The listing builds one solid part. Answer for the finished solid, in the listing's coordinates (mm). Face numbers are marked on the shaded views. A direction names the side the tool comes from. Give positions to 0.01 mm unless a question says otherwise; leave off trailing zeros. Loops run counter-clockwise (first coordinate to the right, second up) from the corner with the lowest first, then second, coordinate; pieces in that order, holes last. Notation, with made-up numbers: (51.5, 31.5) - (75.5, 31.5) arc R19 ccw to (75.5, 63.5) - close; hole circle Ø7 at (-11.75, 51.25). An arc over 180 degrees is marked (long way). Write item = value, one per line. Start each with the question number.
1) Which of the six approach directions +Z, -Z, +X, -X, +Y, -Y give full straight-line access (tool end or side, diameter ignored) to the marked faces 1 and 2?
2) Flat-ended cylindrical pins translate along their axes: P1, Ø3.5, axis at x = 49.5, y = -12.5, coming from the +Z side; P2, Ø2.5, axis at y = -20.5, z = 44.6, coming from the +X side; P3, Ø12, axis at y = -5, z = 23.5, coming from the -X side. Find the tip coordinate at first contact, or state that the pin passes through.
3) The part is cut by section A-A on z = 44.6. Write down the section's boundary in (x, y), plus the area to 3 significant figures.
4) The part is cut by section D-D on y = -20.5. Write down the section's boundary in (x, z).
5) The part is cut by section C-C on y = -12.5. Write down the section's boundary in (x, z), plus the area to 3 significant figures.
6) Consider probe 1 along Y at (x, z) = (57.5, 1); probe 2 along X at (y, z) = (-20.5, 0.9); probe 3 along Y at (x, z) = (101.25, 36.6). Determine where each line is inside the solid, lowest interval first.
7) The part is cut by section B-B on x = 57.5. Write down the section's boundary in (y, z).
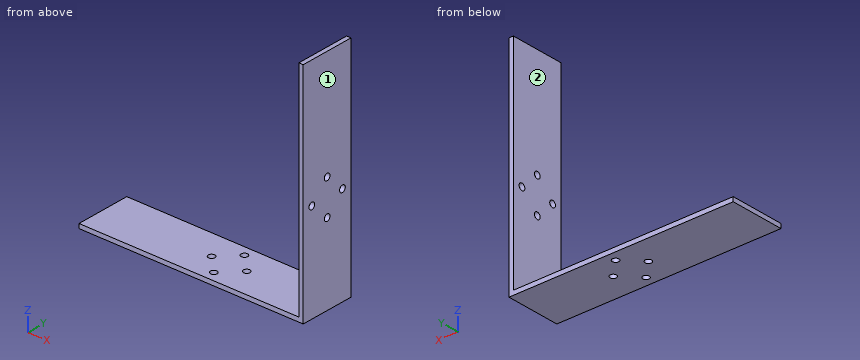
from build123d import *

# Parameters (mm, degrees)
BOSS_EXTRUDE1_DEPTH = 25
SKETCH2_R           = 1.5
CUT_EXTRUDE1_DEPTH  = 11.313708668
SKETCH3_R           = 1.5
CUT_EXTRUDE2_DEPTH  = 25


with BuildPart() as part:
    # Sketch1 → Boss-Extrude1 (new body)
    with BuildSketch(Plane(origin=(0, 0, 0), x_dir=(1, 0, 0), z_dir=(0, 1, 0))):
        Polygon((0, 0), (102.1, 0), (102.1, -102.1), (100.1, -102.1), (100.1, -2), (0, -2), align=None)
    extrude(amount=-BOSS_EXTRUDE1_DEPTH)

    # Sketch2 → Cut-Extrude1 (cut)
    with BuildSketch(Plane(origin=(0, 0, 0), x_dir=(-1, 0, 0), z_dir=(0, 0, -1))):
        with Locations((-65.500000119, -12.5)):
            Circle(SKETCH2_R)
        with Locations((-57.5, -20.500000119)):
            Circle(SKETCH2_R)
        with Locations((-49.499999881, -12.5)):
            Circle(SKETCH2_R)
        with Locations((-57.5, -4.499999881)):
            Circle(SKETCH2_R)
    extrude(amount=-CUT_EXTRUDE1_DEPTH, mode=Mode.SUBTRACT)

    # Sketch3 → Cut-Extrude2 (cut)
    with BuildSketch(Plane(origin=(102.1, 0, 0), x_dir=(0, 0, -1), z_dir=(1, 0, 0))):
        with Locations((-44.6, -4.499999881)):
            Circle(SKETCH3_R)
        with Locations((-36.599999881, -12.5)):
            Circle(SKETCH3_R)
        with Locations((-52.600000119, -12.5)):
            Circle(SKETCH3_R)
        with Locations((-44.6, -20.500000119)):
            Circle(SKETCH3_R)
    extrude(amount=-CUT_EXTRUDE2_DEPTH, mode=Mode.SUBTRACT)


solid = part.part
Answer below:
q1.face_1 = +Z, -Z, +X, +Y, -Y
q1.face_2 = +Z, -X, +Y, -Y
q2.P1 = 2
q2.P2 = through
q2.P3 = 100.1
q3.outline = (100.1, -25) - (102.1, -25) - (102.1, -22) - (100.1, -22) - close; (100.1, -19) - (102.1, -19) - (102.1, -6) - (100.1, -6) - close; (100.1, -3) - (102.1, -3) - (102.1, 0) - (100.1, 0) - close
q3.area = 38.0 mm2
q4.outline = (0, 0) - (56, 0) - (56, 2) - (0, 2) - close; (59, 0) - (102.1, 0) - (102.1, 43.1) - (100.1, 43.1) - (100.1, 2) - (59, 2) - close; (100.1, 46.1) - (102.1, 46.1) - (102.1, 102.1) - (100.1, 102.1) - close
q5.outline = (0, 0) - (48, 0) - (48, 2) - (0, 2) - close; (51, 0) - (64, 0) - (64, 2) - (51, 2) - close; (67, 0) - (102.1, 0) - (102.1, 35.1) - (100.1, 35.1) - (100.1, 2) - (67, 2) - close; (100.1, 38.1) - (102.1, 38.1) - (102.1, 51.1) - (100.1, 51.1) - close; (100.1, 54.1) - (102.1, 54.1) - (102.1, 102.1) - (100.1, 102.1) - close
q5.area = 380 mm2
q6.probe_1 = -25 to -22, -19 to -6, -3 to 0
q6.probe_2 = 0 to 56, 59 to 102.1
q6.probe_3 = -25 to -14, -11 to 0
q7.outline = (-25, 0) - (-22, 0) - (-22, 2) - (-25, 2) - close; (-19, 0) - (-6, 0) - (-6, 2) - (-19, 2) - close; (-3, 0) - (0, 0) - (0, 2) - (-3, 2) - close
